The listing builds one solid part. Answer for the finished solid, in the listing's coordinates (mm). Round coordinates to 2 decimals unless told otherwise and drop trailing zeros. Loops run counter-clockwise (first coordinate to the right, second up) from the corner with the lowest first, then second, coordinate; pieces in that order, holes last. Notation, with made-up numbers: (14.5, 21) - (36.5, 21) arc R29 ccw to (36.5, 59) - close; hole circle Ø8 at (76, 71). An arc over 180 degrees is marked (long way). One line per question, with ' | ' between items. Start each with the question number.
from build123d import *

# Parameters (mm, degrees)
F0_W      = 1625.6
F0_H      = 635
F1_DEPTH  = 127
F1_FACE_W = 1625.6
F1_FACE_H = 127
F2_DEPTH  = 304.8
F3_R      = 50.8


with BuildPart() as f1:
    # F0 (on Top) → F1 (new body)
    with BuildSketch(Plane.XY):
        Rectangle(F0_W, F0_H)
    extrude(amount=F1_DEPTH)

    # F1_face (on face) → F2 (join)
    with BuildSketch(Plane(origin=(0, -317.5, 63.5), x_dir=(1, 0, 0), z_dir=(0, -1, 0))):
        Rectangle(F1_FACE_W, F1_FACE_H)
    extrude(amount=F2_DEPTH)

    # F3
    f3_edges = [f1.edges().sort_by_distance(p)[0] for p in [
        (812.8, -152.4, 127),
        (0, 317.5, 127),
        (-812.8, -152.4, 127),
        (0, -622.3, 127),
        (0, -622.3, 0),
        (812.8, 317.5, 63.5),
        (812.8, -152.4, 0),
        (812.8, -622.3, 63.5),
        (-812.8, 317.5, 63.5),
        (0, 317.5, 0),
        (-812.8, -622.3, 63.5),
        (-812.8, -152.4, 0),
    ]]
    fillet(f3_edges, radius=F3_R)


solid = f1.part
(1) Each of these flat-tipped pins is pushed along its axis until it touches: P1, Ø6, axis at x = -153, z = 44, coming from the -Y side; P2, Ø4, axis at x = 10.5, z = 87, coming from the +Y side; P3, Ø4, axis at x = 378, z = 91.5, coming from the -Y side. Where does it stop, or does it pass through?
(2) Consider L1, parallel to X at y = 110, z = 49; L2, parallel to X at y = -373, z = 47.5; L3, parallel to Y at x = -334, z = 120. Determine where each line is inside the solid, lowest interval first.
(3) Find section B-B on x = 254. Write down the section's boundary in (y, z).
(4) Find section A-A on z = 17.5. Write down the section's boundary in (x, y).
Answer below:
1) P1: y = -622.16 | P2: y = 316.73 | P3: y = -620.53
2) L1: -812.77 to 812.77 | L2: -812.69 to 812.69 | L3: -597.23 to 292.43
3) outline: (-622.3, 50.8) arc R50.8 ccw to (-571.5, 0) - (266.7, 0) arc R50.8 ccw to (317.5, 50.8) - (317.5, 76.2) arc R50.8 ccw to (266.7, 127) - (-571.5, 127) arc R50.8 ccw to (-622.3, 76.2) - close
4) outline: (-800.36, -571.5) arc R38.36 ccw to (-762, -609.86) - (762, -609.86) arc R38.36 ccw to (800.36, -571.5) - (800.36, 266.7) arc R38.36 ccw to (762, 305.06) - (-762, 305.06) arc R38.36 ccw to (-800.36, 266.7) - close
